Part print with two shaded views. Sizes in mm from the minimum x, y, z corner. A direction names the side the tool comes from. Round coordinates to 2 decimals unless told otherwise and drop trailing zeros. Order: outer loops, then holes, each group sorted by start corner. A loop starts at its lowest first (then second) coordinate and runs counter-clockwise, first axis right, second up. Notation, with made-up numbers: (81, 57.5) -> (85, 57.5) arc R34 ccw to (85, 91.5) -> close; hole circle Ø4 at (-22.5, 44). An arc over 180 degrees is marked (long way). Use a Markdown table: item, result. Add a question column.
Item 1: Slice it at B-B, the plane x = 6. Give the cut face in (y, z), plus the area to 3 significant figures.
Item 2: Two-plate mould, pull along X, no slides. Class the marked faces 1, 2 and 3: released by +X, released by -X, zero draft, split by the parting line, or undercut.
Item 3: Probe L1, parallel to Y at x = 6, z = 5.75; L2, parallel to X at y = 13.35, z = 4; L3, parallel to Y at x = 9.25, z = 3. List the from-to ranges inside material, lowest first.
Item 4: 3-axis set-ups, long thin cutter, end or side, ignore diameter. For the marked faces 4, 5 and 6: which of +Z, -Z, +X, -X, +Y, -Y reach the whole face in a straight line?
Item 5: Slice it at D-D, the plane y = 8. Give the cut face in (x, z).
Item 6: Slice it at C-C, the plane y = 11.5. Give the cut face in (x, z).
Item 7: Pin check, flat tips, straight feed: pin 1 (0.9 mm diameter, centred on y = 13.5, z = 3.5, fed in from -X); pin 2 (0.9 mm diameter, centred on y = 13.5, z = 4.5, fed in from +X); pin 3 (0.5 mm diameter, centred on x = 10.5, z = 2.5, fed in from +Y). Stop position of each tip, or through.
Item 8: Slice it at A-A, the plane z = 1.5. Give the cut face in (x, y).
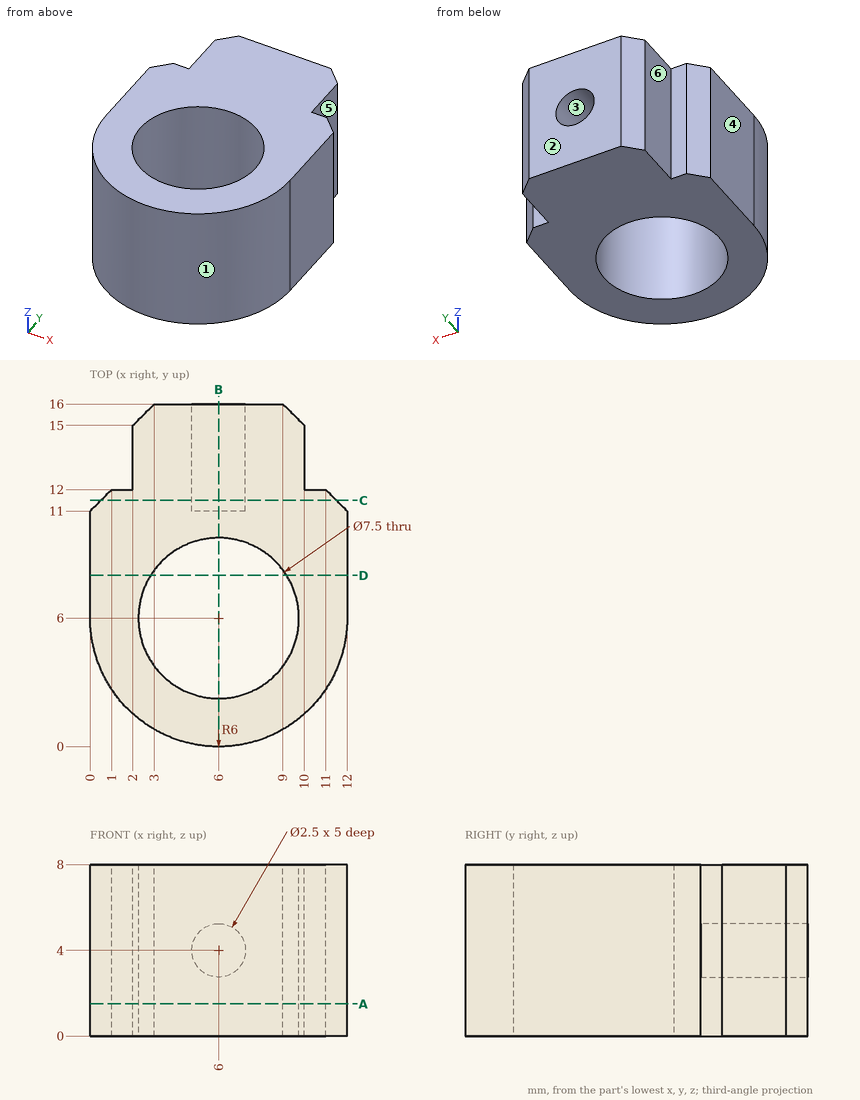
Check sheet entries:
| question | item | result |
|---|---|---|
| 1 | outline | (0, 0) -> (2.25, 0) -> (2.25, 8) -> (0, 8) -> close; (9.75, 0) -> (16, 0) -> (16, 2.75) -> (11, 2.75) -> (11, 5.25) -> (16, 5.25) -> (16, 8) -> (9.75, 8) -> close |
| 1 | area | 55.5 mm2 |
| 2 | face 1 | split by the parting line |
| 2 | face 2 | zero draft |
| 2 | face 3 | undercut |
| 3 | L1 | 0 to 2.25, 9.75 to 16 |
| 3 | L2 | 2 to 4.75, 7.25 to 10 |
| 3 | L3 | 0.96 to 4.13, 7.87 to 15.75 |
| 4 | face 4 | +Z, -Z, -X, +Y, -Y |
| 4 | face 5 | +Z, -Z, +X, +Y |
| 4 | face 6 | +Z, -Z, -X, +Y |
| 5 | outline | (0, 0) -> (2.83, 0) -> (2.83, 8) -> (0, 8) -> close; (9.17, 0) -> (12, 0) -> (12, 8) -> (9.17, 8) -> close |
| 6 | outline | (0.5, 0) -> (11.5, 0) -> (11.5, 8) -> (0.5, 8) -> close; hole circle Ø2.5 at (6, 4) |
| 7 | pin 1 | x = 2 |
| 7 | pin 2 | x = 10 |
| 7 | pin 3 | y = 12 |
| 8 | outline | (0, 6) arc R6 ccw to (12, 6) -> (12, 11) -> (11, 12) -> (10, 12) -> (10, 15) -> (9, 16) -> (3, 16) -> (2, 15) -> (2, 12) -> (1, 12) -> (0, 11) -> close; hole circle Ø7.5 at (6, 6) |
